Check sheet for the modelled part. Datum: model origin and axes. Units: mm. A direction names the side the tool comes from. Round coordinates to 2 decimals unless told otherwise and drop trailing zeros. Loops run counter-clockwise (first coordinate to the right, second up) from the corner with the lowest first, then second, coordinate; pieces in that order, holes last. Notation, with made-up numbers: (-40, 71) -> (-5, 71) arc R16 ccw to (-5, 97) -> close; hole circle Ø3 at (-28.75, -25). An arc over 180 degrees is marked (long way). One line per item, written item: value. Start each with the question number.
1. Set-up check for faces 1 (the face through (0, 0, 0)), 2 (the face through (-0.7, -3.1, 51.7)): record each of +Z, -Z, +X, -X, +Y, -Y from which the full face is reachable in a straight line by a thin tool's end or side.
2. Cross-section at D-D on z = 9.5. Record the cut outline in (x, y).
3. Material ranges on L1, parallel to Z at x = 24, y = -6; L2, parallel to Z at x = 2, y = 10.5; L3, parallel to X at y = 7, z = 5, recorded low to high.
4. Cross-section at C-C on z = 37. Record the cut outline in (x, y).
5. Go/stop test with flat-tipped pins: pin 1 (1 mm diameter, centred on x = -9, y = -8.5, fed in from +Z); pin 2 (3 mm diameter, centred on x = 20.5, y = 4, fed in from -Z); pin 3 (6 mm diameter, centred on y = -5, z = 53, fed in from -X); pin 4 (5 mm diameter, centred on x = -5, y = -19, fed in from +Z). Record where each tip stops, or that it passes through.
6. Cross-section at A-A on y = 0. Record the cut outline in (x, z).
from build123d import *

# Parameters (mm, degrees)
F2_SIZE = 1.25


with BuildPart() as f1:
    # F0 (on Front) → F1 (revolve)
    with BuildSketch(Plane.XZ):
        with BuildLine():
            Line((0, 85.55), (0, 0))
            Line((0, 0), (26.67, 0))
            Line((26.67, 0), (26.67, 1.27))
            Line((26.67, 1.27), (23.975923, 3.964077))
            ThreePointArc((23.975923, 3.964077), (9.828048, 5.577479), (3.18, 18.169894))
            Line((3.18, 18.169894), (3.18, 85.55))
            Line((3.18, 85.55), (0, 85.55))
        make_face()
    revolve(axis=Axis((0, 0, 42.775), (0, 0, 1)))

    # F2
    f2_edges = [f1.edges().sort_by_distance(p)[0] for p in [
        (-3.18, 0, 85.55),
    ]]
    chamfer(f2_edges, length=F2_SIZE)


solid = f1.part
Taken from the geometry:
1. face 1: -Z, +X, -X, +Y, -Y
1. face 2: +Z
2. outline: circle Ø11.77 at (0, 0)
3. L1: z = 0 to 3.2
3. L2: z = 0 to 5.03
3. L3: x = -8.15 to 8.15
4. outline: circle Ø6.36 at (0, 0)
5. pin 1: stops at z = 4.4
5. pin 2: stops at z = 0
5. pin 3: stops at x = -2.47
5. pin 4: stops at z = 3.38
6. outline: (-26.67, 0) -> (26.67, 0) -> (26.67, 1.27) -> (23.98, 3.96) arc R15.25 cw to (3.18, 18.17) -> (3.18, 84.3) -> (1.93, 85.55) -> (-1.93, 85.55) -> (-3.18, 84.3) -> (-3.18, 18.17) arc R15.25 cw to (-23.98, 3.96) -> (-26.67, 1.27) -> close
